Autodesk Inventor part; units mm, degrees
ref_plane "YZ Plane" through (0, 0, 0) normal (1, 0, 0) x (0, 1, 0)
ref_plane "XZ Plane" through (0, 0, 0) normal (0, 1, 0) x (-1, 0, 0)
ref_plane "XY Plane" through (0, 0, 0) normal (0, 0, 1) x (1, 0, 0)
sketch "Sketch1" plane through (0, 0, 0) normal (0, 0, 1) x (1, 0, 0)
  line L0 (-5.7, 0) -> (-5.7, -5.7)
  line L1 (-5.7, -5.7) -> (0, -5.7)
  line L2 (0, 5.7) -> (-5.7, 5.7)
  line L3 (-5.7, 5.7) -> (-5.7, 0)
  line L4 (0, 4.1) -> (-4.1, 4.1)
  line L5 (-4.1, 4.1) -> (-4.1, -4.1)
  line L6 (-4.1, -4.1) -> (0, -4.1)
  line L7 (3.9, -5.7) -> (0, -5.7)
  line L8 (3.9, 5.7) -> (0, 5.7)
  line L9 (3.9, 5.7) -> (5.5, 5.7)
  line L10 (3.9, -5.7) -> (5.5, -5.7)
  line L11 (5.5, 4.1) -> (0, 4.1)
  line L12 (5.5, -4.1) -> (0, -4.1)
  line L13 (0, 0) -> (4.1, 0)
  line L14 (4.1, 0) -> (5.7, 0)
  line L15 (5.7, 0) -> (5.7, 5.7)
  line L16 (5.7, 5.7) -> (5.5, 5.7)
  line L17 (5.5, 4.1) -> (5.7, 4.1)
  line L18 (5.7, 0) -> (5.7, -5.7)
  line L19 (5.7, -5.7) -> (5.5, -5.7)
  line L20 (5.5, -4.1) -> (5.7, -4.1)
  dimension "d22" = 4.1
  dimension "d23" = 1.6
extrude "Extrusion1" add sketch "Sketch1" against normal blind 15 contours L3 L2 L8 L9 L16 L15 L17 L11 L4 L5 L6 L12 L20 L18 L19 L10 L7 L1 L0
sketch "Sketch2" plane through (-5.7, 5.7, 0) normal (0, 1, 0) x (1, 0, 0)
  line L0 (5.7, 0) -> (5.7, 4.2)
  circle A0 centre (5.7, 4.2) radius 2.15
  dimension "d10" = 4.2
  dimension "d11" = 4.3
extrude "Extrusion2" cut sketch "Sketch2" against normal blind 15
sketch "Sketch3" plane through (0, 0, 0) normal (0, 0, 1) x (1, 0, 0)
  point P0 (0, 0)
sketch "Sketch4" plane through (0, 0, 0) normal (0, 0, 1) x (1, 0, 0)
  point P0 (5.5, 5.7)
sketch "Sketch5" plane through (0, 0, 0) normal (0, 0, 1) x (1, 0, 0)
  line L0 (5.7, 4.1) -> (5.7, 0)
  line L1 (5.7, 0) -> (5.7, 24)
  line L2 (5.7, 0) -> (5.7, -24)
  line L3 (5.7, -25.6) -> (4.1, -25.6)
  line L4 (5.7, -5.7) -> (-5.7, -5.7)
  line L5 (4.1, -5.7) -> (4.1, -25.6)
  line L6 (5.7, 25.6) -> (4.1, 25.6)
  line L7 (4.1, 25.6) -> (4.1, 5.7)
  line L8 (5.7, 5.7) -> (-5.7, 5.7)
  line L9 (5.7, 25.6) -> (18.7, 25.6)
  line L10 (18.7, 25.6) -> (18.7, 24)
  line L11 (18.7, 24) -> (5.7, 24)
  line L12 (5.7, -25.6) -> (18.7, -25.6)
  line L13 (18.7, -25.6) -> (18.7, -24)
  line L14 (18.7, -24) -> (5.7, -24)
  line L15 (4.1, 5.7) -> (4.1, -5.7)
  line L16 (5.7, -4.1) -> (-4.1, -4.1)
  line L17 (4.1, 5.7) -> (5.7, 5.7)
  line L18 (4.1, 4.1) -> (5.7, 4.1)
  line L19 (4.1, -4.1) -> (5.7, -4.1)
  line L20 (4.1, -5.7) -> (5.7, -5.7)
  point P0 (0, 0)
extrude "Extrusion3" add sketch "Sketch5" against normal blind 15 contours L8 L7 L6 L9 L10 L11 L1 | L2 L14 L13 L12 L3 L5 L4
sketch "Sketch6" plane through (0, 0, 0) normal (0, 0, 1) x (1, 0, 0)
  line L0 (18.7, -25.6) -> (4.1, -25.6)
  line L1 (4.1, -25.6) -> (4.1, 4.1)
  line L2 (5.7, 4.1) -> (-4.1, 4.1)
  line L3 (5.7, -4.1) -> (5.7, -24)
  line L4 (5.7, 4.1) -> (5.7, -24)
  line L5 (4.1, -25.6) -> (18.7, -25.6)
  line L6 (18.7, -24) -> (18.7, -25.6)
  line L7 (18.7, -24) -> (5.7, -24)
  line L8 (18.7, -24) -> (5.7, -24)
  line L9 (5.7, 4.1) -> (5.7, 24)
  line L10 (5.7, 4.1) -> (5.7, 24)
  line L11 (5.7, 24) -> (18.7, 24)
  line L12 (18.7, 25.6) -> (4.1, 25.6)
  line L13 (18.7, 24) -> (18.7, 25.6)
  line L14 (18.7, 25.6) -> (18.7, 24)
  line L15 (18.7, 25.6) -> (4.1, 25.6)
  line L16 (4.1, 4.1) -> (4.1, 25.6)
  line L17 (4.1, 5.7) -> (-5.7, 5.7)
  point P0 (0, 0)
extrude "Extrusion4" add sketch "Sketch6" along normal blind 18.6
sketch "Sketch7" plane through (5.7, 4.1, -15) normal (1, 0, 0) x (0, 0, -1)
  line L0 (0, -28.1) -> (-33.6, -28.1)
  line L1 (-33.6, -28.1) -> (-33.6, 19.9)
  line L2 (-33.6, -28.1) -> (-33.6, 19.9)
  line L3 (-33.6, 19.9) -> (-32, 19.9)
  line L4 (0, 19.9) -> (-33.6, 19.9)
  line L5 (-32, 19.9) -> (-32, -28.1)
  line L6 (-32, -28.1) -> (-33.6, -28.1)
  point P0 (-15, -4.1)
  dimension "d35" = 1.6
extrude "Extrusion5" add sketch "Sketch7" along normal blind 13
sketch "Sketch8" plane through (5.7, -24, -15) normal (1, 0, 0) x (0, 0, -1)
  line L0 (0, 0) -> (0, -1.6)
  line L1 (-8.4022, 0) -> (-11.0502, 0)
  line L2 (-32, 0) -> (0, 0)
  line L3 (-11.0502, 0) -> (-10.0022, 0)
  line L4 (-10.0022, 0) -> (-10.0022, 18.3)
  line L5 (0, 18.3) -> (-15, 18.3)
  line L6 (0, 49.6) -> (-33.6, 49.6)
  line L7 (-8.4022, 49.6) -> (-10.0022, 49.6)
  line L8 (-15, 29.7) -> (0, 29.7)
  line L9 (-10.0022, 29.7) -> (-10.0022, 49.6)
  line L10 (-10.0022, 0) -> (-10.0022, 18.3)
  line L11 (-10.0022, 29.7) -> (-10.0022, 48)
  line L12 (-32, 48) -> (0, 48)
  line L13 (-10.0022, 0) -> (-8.4022, 0)
  line L14 (-8.4022, 0) -> (-8.4022, 18.3)
  line L15 (-8.4022, 29.7) -> (-8.4022, 48)
  line L16 (-10.0022, 18.3) -> (-8.4022, 18.3)
  line L17 (-10.0022, 29.7) -> (-8.4022, 29.7)
  line L18 (-10.0022, 48) -> (-8.4022, 48)
  line L19 (-10.0022, 0) -> (-8.4022, 0)
  point P0 (-15, 24)
  dimension "d38" = 1.6
extrude "Extrusion6" add sketch "Sketch8" along normal blind 8
sketch "Sketch9" plane through (5.7, 24, -15) normal (0, -1, 0) x (1, 0, 0)
  line L0 (13, 0) -> (0, 0)
  line L1 (13, 0) -> (13, 1.6)
  line L2 (13, 32) -> (13, 0)
  line L3 (13, 1.6) -> (0, 1.6)
  line L4 (0, 0) -> (0, 8.4022)
  line L5 (0, 0) -> (0, 1.6)
  line L6 (-1.6, 0) -> (13, 0)
  line L7 (0, 0) -> (13, 0)
  point P0 (-5.7, 15)
  dimension "d41" = 1.6
extrude "Extrusion7" add sketch "Sketch9" along normal blind 48
sketch "Sketch10" plane through (18.7, -25.6, -15) normal (1, 0, 0) x (0, 0, -1)
  point P0 (-15, 25.6)
sketch "Sketch11" plane through (5.7, 24, 17) normal (0, -1, 0) x (1, 0, 0)
  line L0 (8, -23.5978) -> (8, -26.9978)
  line L1 (0, -30.4) -> (13, -30.4)
  circle A0 centre (8, -26.9978) radius 2.05
  point P0 (-5.7, -17)
  dimension "d44" = 3.4
  dimension "d45" = 4.1
extrude "Extrusion8" cut sketch "Sketch11" along normal blind 59
extrude "Extrusion9" cut sketch "Sketch11" against normal blind 18
Geometry: final body of the model. Coordinates: model frame, mm. A direction names the side the tool comes from. Round coordinates to 2 decimals unless told otherwise and drop trailing zeros. Write each loop counter-clockwise with the first axis right and the second up, starting at its lowest first coordinate (ties: lowest second). Pieces come first, ordered by that corner, then holes.
Item 1: Section query A-A (x = 0). Return loops of the section in (y, z).
Item 2: Section query B-B (z = -4.2). Return loops of the section in (x, y), plus the area to 3 significant figures.
Item 3: Section query C-C (x = 3.5). Return loops of the section in (y, z).
Item 4: Mould query, pull axis X, two halves, no side actions, for faces 1 (the face through (18.7, 0, -14)), 2 (the face through (12, 0, -13.4)), 3 (the face through (13.433, 24.789, -7.965)). Classes: +X half, -X half, draft (parallel to the pull), parting line (faces both ways), or undercut.
Item 5: Pin query (flat end, axial travel): P1, Ø5, axis at x = -1, z = -7.5, coming from the +Y side; P2, Ø1, axis at y = -19.5, z = 3.5, coming from the +X side; P3, Ø4, axis at y = -1, z = -11, coming from the +X side; P4, Ø2.5, axis at x = 13.7, z = -10, coming from the +Y side. Return the tip coordinate at first contact, or that it passes through.
Item 6: Section query D-D (y = 1.5). Return loops of the section in (x, z).
Item 7: Set-up query: faces 4 (the face through (5, 0, 0)), 5 (the face through (-1, 5.7, -7)), 6 (the face through (12, 0, 17)), 7 (the face through (-1, -5.7, -7)), 8 (the face through (1, -4.1, -7)). Return all of +Z, -Z, +X, -X, +Y, -Y with unobstructed straight access to the full face (end or side cutting, diameter ignored); none if empty.
Item 8: Material intervals for L1, parallel to Y at x = 4.25, z = -12; L2, parallel to Y at x = 6.5, z = 0.5; L3, parallel to Z at x = 0, y = 4.8, sorted ascending.
Completed:
1. outline: (-5.7, -15) - (-4.1, -15) - (-4.1, -6.35) - (-5.7, -6.35) - close; (-5.7, -2.05) - (-4.1, -2.05) - (-4.1, 0) - (-5.7, 0) - close; (4.1, -15) - (5.7, -15) - (5.7, -6.35) - (4.1, -6.35) - close; (4.1, -2.05) - (5.7, -2.05) - (5.7, 0) - (4.1, 0) - close
2. outline: (-5.7, -5.7) - (-2.15, -5.7) - (-2.15, -4.1) - (-4.1, -4.1) - (-4.1, 4.1) - (-2.15, 4.1) - (-2.15, 5.7) - (-5.7, 5.7) - close; (2.15, -5.7) - (4.1, -5.7) - (4.1, -25.6) - (18.7, -25.6) - (18.7, -24) - (5.7, -24) - (5.7, -4.1) - (2.15, -4.1) - close; (2.15, 4.1) - (5.7, 4.1) - (5.7, 24) - (18.7, 24) - (18.7, 25.6) - (4.1, 25.6) - (4.1, 5.7) - (2.15, 5.7) - close
2. area: 141 mm2
3. outline: (-5.7, -15) - (-4.1, -15) - (-4.1, 0) - (-5.7, 0) - close; (4.1, -15) - (5.7, -15) - (5.7, 0) - (4.1, 0) - close
4. face 1: +X half
4. face 2: draft
4. face 3: undercut
5. P1: stops at y = 5.7
5. P2: stops at x = 5.7
5. P3: stops at x = -4.1
5. P4: passes through
6. outline: (-5.7, -15) - (-4.1, -15) - (-4.1, 0) - (-5.7, 0) - close; (4.1, 0) - (5.7, 0) - (5.7, 17) - (18.7, 17) - (18.7, 18.6) - (4.1, 18.6) - close; (5.7, -15) - (18.7, -15) - (18.7, -13.4) - (5.7, -13.4) - close
7. face 4: -Z, +X
7. face 5: +Z, -Z, -X, +Y
7. face 6: +X
7. face 7: +Z, -Z, -X, -Y
7. face 8: -Z
8. L1: y = -25.6 to -4.1, 4.1 to 25.6
8. L2: y = -25.6 to -24, 24 to 25.6
8. L3: z = -15 to -6.35, -2.05 to 0
